from build123d import *

# Parameters (mm, degrees)
SKETCH_1_W          = 130
SKETCH_1_H          = 25
EXTRUDE_1_DEPTH     = 4.5
SKETCH_2_R          = 5
EXTRUDE_2_DEPTH     = 57
SKETCH_3_R          = 8
EXTRUDE_3_DEPTH     = 21
SKETCH_4_R          = 6
EXTRUDE_4_DEPTH     = 47
CUT_EXTRUDE_1_REACH = 96.896
SKETCH_5_R          = 2


with BuildPart() as part:
    # Эскиз1 → Бобышка-Вытянуть1 (new body)
    with BuildSketch(Plane(origin=(0, 0, 0), x_dir=(1, 0, 0), z_dir=(0, 1, 0))):
        Rectangle(SKETCH_1_W, SKETCH_1_H)
    extrude(amount=EXTRUDE_1_DEPTH)

    # Эскиз2 → Бобышка-Вытянуть2 (add)
    with BuildSketch(Plane(origin=(0, 4.5, 0), x_dir=(1, 0, 0), z_dir=(0, 1, 0))):
        with Locations(Location((48.4, 0, 0), (0, 0, 90))):
            Circle(SKETCH_2_R)
    extrude(amount=EXTRUDE_2_DEPTH)

    # Эскиз3 → Бобышка-Вытянуть3 (add)
    with BuildSketch(Plane.XZ):
        with Locations(Location((-50, 0, 0), (0, 0, 90))):
            Circle(SKETCH_3_R)
    extrude(amount=EXTRUDE_3_DEPTH)

    # Эскиз4 → Бобышка-Вытянуть4 (add)
    with BuildSketch(Plane.XZ.offset(21)):
        with Locations(Location((-50, 0, 0), (0, 0, 270))):
            Circle(SKETCH_4_R)
    extrude(amount=EXTRUDE_4_DEPTH)

    # Эскиз5 → Вырез-Вытянуть1 (cut, up to next)
    with BuildSketch(Plane.XZ, mode=Mode.PRIVATE) as cut_extrude_1_sk1:
        with Locations(Location((0, 7, 0), (0, 0, 270))):
            Circle(SKETCH_5_R)
    cut_extrude_1_tool1 = extrude(cut_extrude_1_sk1.sketch, amount=-CUT_EXTRUDE_1_REACH, mode=Mode.PRIVATE) & part.part
    # Эскиз5 → Вырез-Вытянуть1 (cut, up to next)
    with BuildSketch(Plane.XZ, mode=Mode.PRIVATE) as cut_extrude_1_sk2:
        with Locations(Location((0, -7, 0), (0, 0, 270))):
            Circle(SKETCH_5_R)
    cut_extrude_1_tool2 = extrude(cut_extrude_1_sk2.sketch, amount=-CUT_EXTRUDE_1_REACH, mode=Mode.PRIVATE) & part.part
    add(cut_extrude_1_tool1.solids().sort_by_distance((0, 0, 7))[0], mode=Mode.SUBTRACT)
    add(cut_extrude_1_tool2.solids().sort_by_distance((0, 0, -7))[0], mode=Mode.SUBTRACT)


solid = part.part
Work out the finished part from the listing and answer in its coordinate system (mm). A direction names the side the tool comes from. Round coordinates to 2 decimals unless told otherwise and drop trailing zeros. Write each loop counter-clockwise with the first axis right and the second up, starting at its lowest first coordinate (ties: lowest second). Pieces come first, ordered by that corner, then holes. Notation, with made-up numbers: (72.25, 24) - (112.25, 24) arc R21 ccw to (112.25, 32) - close; hole circle Ø9 at (45.25, 77). An arc over 180 degrees is marked (long way). Answer in a Markdown table with one row per item. Add a question column.
1. The mould has two halves that part along X. Classify faces 1 (the cylindrical face through (0, 2, -5)), 2 (the flat face through (-65, 2, 0)), 3 (the flat face through (-1, 4.5, 0)): +X half, -X half, draft (parallel to the pull), parting line (faces both ways), or undercut.
2. For faces 4 (the flat face through (65, 2, 0)), 5 (the cylindrical face through (53.28, 32.6, 1.08)), 6 (the cylindrical face through (-57.932, -10.353, -1.041)), determine the directions among +Z, -Z, +X, -X, +Y, -Y from which every point of the face is accessible in a straight line to the end or side of a thin tool.
3. A cutting plane is placed at D-D, the plane y = 15. Determine the outline of the cut face in (x, z).
4. A cutting plane is placed at C-C, the plane z = 0. Determine the outline of the cut face in (x, y).
5. Given pin 1 (5 mm diameter, centred on x = 0, z = 7, fed in from +Y); pin 2 (10 mm diameter, centred on x = 45, y = 17.5, fed in from -Z); pin 3 (6 mm diameter, centred on x = -28.5, z = -0.5, fed in from -Y), each flat-ended and moving along its own axis, determine where each tip first touches the part or whether it passes through.
6. Find the intervals of material crossed by line 1 along X through (y, z) = (3.4, 7); line 2 along Y through (x, z) = (45.5, -2.25); line 3 along Y through (x, z) = (-53, 3), in increasing order. Write a range as from..to.
7. A cutting plane is placed at B-B, the plane x = 48.4. Determine the outline of the cut face in (y, z), and give its area (4 significant figures).
8. A cutting plane is placed at A-A, the plane x = 0. Determine the outline of the cut face in (y, z), and give its area (3 significant figures).
Worked out:
| question | item | result |
|---|---|---|
| 1 | face 1 | undercut |
| 1 | face 2 | -X half |
| 1 | face 3 | draft |
| 2 | face 4 | +Z, -Z, +X, +Y, -Y |
| 2 | face 5 | +Y |
| 2 | face 6 | -Y |
| 3 | outline | circle Ø10 at (48.4, 0) |
| 4 | outline | (-65, 0) - (-58, 0) - (-58, -21) - (-56, -21) - (-56, -68) - (-44, -68) - (-44, -21) - (-42, -21) - (-42, 0) - (65, 0) - (65, 4.5) - (53.4, 4.5) - (53.4, 61.5) - (43.4, 61.5) - (43.4, 4.5) - (-65, 4.5) - close |
| 5 | pin 1 | y = 4.5 |
| 5 | pin 2 | z = -5 |
| 5 | pin 3 | y = 0 |
| 6 | line 1 | -65..-2, 2..65 |
| 6 | line 2 | 0..61.5 |
| 6 | line 3 | -68..4.5 |
| 7 | outline | (0, -12.5) - (4.5, -12.5) - (4.5, -5) - (61.5, -5) - (61.5, 5) - (4.5, 5) - (4.5, 12.5) - (0, 12.5) - close |
| 7 | area | 682.5 mm^2 |
| 8 | outline | (0, -12.5) - (4.5, -12.5) - (4.5, -9) - (0, -9) - close; (0, -5) - (4.5, -5) - (4.5, 5) - (0, 5) - close; (0, 9) - (4.5, 9) - (4.5, 12.5) - (0, 12.5) - close |
| 8 | area | 76.5 mm^2 |
